```python
from build123d import *

# Parameters (mm, degrees)
SKETCH4_R           = 10
BOSS_EXTRUDE1_DEPTH = 80
SKETCH5_W           = 40
SKETCH5_H           = 20
CUT_EXTRUDE1_DEPTH  = 139.564064606
FILLET1_R           = 3
CHAMFER1_SIZE       = 5
FILLET2_R           = 5
FILLET4_R           = 5
CHAMFER3_SIZE       = 5
FILLET5_R           = 2
FILLET6_R           = 2
CHAMFER4_SIZE       = 5
CHAMFER5_SIZE       = 5


with BuildPart() as part:
    # Sketch4 → Boss-Extrude1 (new body)
    with BuildSketch(Plane(origin=(0, 0, 0), x_dir=(0, 0, -1), z_dir=(1, 0, 0))):
        Polygon((0, 0), (-80, 0), (-80, 40), (-40, 40), (-40, 80), (0, 80), align=None)
        with Locations((-20, 20)):
            Circle(SKETCH4_R, mode=Mode.SUBTRACT)
    extrude(amount=BOSS_EXTRUDE1_DEPTH)

    # Sketch5 → Cut-Extrude1 (cut, through all)
    with BuildSketch(Plane.XZ):
        with Locations((40, 70)):
            Rectangle(SKETCH5_W, SKETCH5_H)
    extrude(amount=-CUT_EXTRUDE1_DEPTH, mode=Mode.SUBTRACT)

    # Fillet1
    fillet1_edges = [part.edges().sort_by_distance(p)[0] for p in [
        (80, 20, 80),
        (0, 20, 80),
    ]]
    fillet(fillet1_edges, radius=FILLET1_R)

    # Chamfer1
    chamfer1_edges = [part.edges().sort_by_distance(p)[0] for p in [
        (20, 20, 80),
        (60, 20, 80),
    ]]
    chamfer(chamfer1_edges, length=CHAMFER1_SIZE)

    # Fillet2
    fillet2_edges = [part.edges().sort_by_distance(p)[0] for p in [
        (20, 20, 60),
        (60, 20, 60),
    ]]
    fillet(fillet2_edges, radius=FILLET2_R)

    # Fillet4
    fillet4_edges = [part.edges().sort_by_distance(p)[0] for p in [
        (40, 40, 40),
    ]]
    fillet(fillet4_edges, radius=FILLET4_R)

    # Chamfer3
    chamfer3_edges = [part.edges().sort_by_distance(p)[0] for p in [
        (40, 80, 40),
    ]]
    chamfer(chamfer3_edges, length=CHAMFER3_SIZE)

    # Fillet5
    fillet5_edges = [part.edges().sort_by_distance(p)[0] for p in [
        (0, 20, 30),
    ]]
    fillet(fillet5_edges, radius=FILLET5_R)

    # Fillet6
    fillet6_edges = [part.edges().sort_by_distance(p)[0] for p in [
        (80, 20, 30),
    ]]
    fillet(fillet6_edges, radius=FILLET6_R)

    # Chamfer4
    chamfer4_edges = [part.edges().sort_by_distance(p)[0] for p in [
        (80, 40, 0),
    ]]
    chamfer(chamfer4_edges, length=CHAMFER4_SIZE)

    # Chamfer5
    chamfer5_edges = [part.edges().sort_by_distance(p)[0] for p in [
        (0, 40, 0),
    ]]
    chamfer(chamfer5_edges, length=CHAMFER5_SIZE)


solid = part.part
```
For this review, take the finished solid that the model builds, in its own axes (mm). A direction names the side the tool comes from. Coordinates: 2 decimals unless noted, no trailing zeros. Order: outer loops, then holes, each group sorted by start corner. A loop starts at its lowest first (then second) coordinate and runs counter-clockwise, first axis right, second up. Notation, with made-up numbers: (62.5, 59) - (110.5, 59) arc R26 ccw to (110.5, 78) - close; hole circle Ø1 at (8.25, -32). An arc over 180 degrees is marked (long way). Answer as a JSON object with one key per item and string values. Group by question number.
1. We need section C-C on y = 72. State the section outline as (x, z) points, then the cut area to 4 significant figures.
2. We need section D-D on x = 18.5. State the section outline as (y, z) points.
3. For probe 1 along X at (y, z) = (20, 74); probe 2 along Y at (x, z) = (28, 20); probe 3 along Y at (x, z) = (12, 73), list the stretches that pass through material, from the lowest coordinate up.
4. We need section B-B on x = 69. State the section outline as (y, z) points, then the cut area to 3 significant figures.
5. The part is to be moulded in two halves that separate along Z. For faces 1 (the cylindrical face through (39.47, 23, 10.46)), 2 (the cylindrical face through (41, 41, 42)), 3 (the flat face through (39, 40, 59)), say which applies: pulls with the +Z half, pulls with the -Z half, needs draft (parallel to the pull), parting line crosses it, or undercut.
6. For faces 4 (the flat face through (62, 20, 77)), 5 (the flat face through (71, 20, 80)), list the 3-axis set-ups (+Z, -Z, +X, -X, +Y, -Y) from which the entire face can be reached by the end or side of a thin tool; tool diameter is ignored.
7. Clearance check with flat-ended pins moving along their axes: P1, Ø18, axis at y = 20, z = 20, coming from the -X side; P2, Ø9, axis at x = 40, y = 22.5, coming from the +Z side; P3, Ø1.5, axis at x = 49.5, z = 46, coming from the +Y side. State where each tip first meets the part, or that it passes through.
8. We need section A-A on z = 20. State the section outline as (x, y) points, then the cut area to 3 significant figures.
Final values:
{
 "1": {"outline": "(0, 5) - (5, 0) - (75, 0) - (80, 5) - (80, 40) - (0, 40) - close", "area": "3,175 mm²"},
 "2": {"outline": "(0, 0) - (80, 0) - (80, 35) - (75, 40) - (45, 40) arc R5 cw to (40, 45) - (40, 76.5) - (0, 76.5) - close; hole circle Ø20 at (20, 20)"},
 "3": {"probe 1": "0 to 20, 60 to 80", "probe 2": "0 to 10, 30 to 80", "probe 3": "0 to 40"},
 "4": {"outline": "(0, 0) - (80, 0) - (80, 35) - (75, 40) - (45, 40) arc R5 cw to (40, 45) - (40, 80) - (0, 80) - close; hole circle Ø20 at (20, 20)", "area": "4,480 mm²"},
 "5": {"face 1": "undercut", "face 2": "pulls with the +Z half", "face 3": "needs draft"},
 "6": {"face 4": "+Z, +Y, -Y", "face 5": "+Z, +X, -X, +Y, -Y"},
 "7": {"P1": "through", "P2": "z = 60", "P3": "y = 40"},
 "8": {"outline": "(0, 0) - (80, 0) - (80, 8) arc R2 ccw to (78, 10) - (2, 10) arc R2 ccw to (0, 8) - close; (0, 32) arc R2 ccw to (2, 30) - (78, 30) arc R2 ccw to (80, 32) - (80, 80) - (0, 80) - close", "area": "4,800 mm²"}
}
